Autodesk Inventor part; units mm, degrees
ref_plane "YZ Plane" through (0, 0, 0) normal (1, 0, 0) x (0, 1, 0)
ref_plane "XZ Plane" through (0, 0, 0) normal (0, 1, 0) x (-1, 0, 0)
ref_plane "XY Plane" through (0, 0, 0) normal (0, 0, 1) x (1, 0, 0)
sketch "Sketch1" plane through (0, 0, 0) normal (0, 0, 1) x (1, 0, 0)
  line L0 (-50, 30) -> (-50, 47.5)
  line L1 (50, 30) -> (50, 47.5)
  line L2 (-18.1144, 47.5) -> (0, 40)
  line L3 (0, 40) -> (18.1144, 47.5)
  line L4 (-100, 30) -> (-50, 30)
  line L5 (50, 30) -> (100, 30)
  line L6 (0, 40) -> (0, 46.5) construction
  line L7 (-18.1144, 47.5) -> (-50, 47.5)
  line L8 (18.1144, 47.5) -> (50, 47.5)
  line L9 (-100, 30) -> (-100, 0)
  line L10 (100, 0) -> (100, 30)
  line L11 (-100, 0) -> (0, 0)
  line L12 (0, 0) -> (100, 0)
  dimension "d90" = 17.5
  dimension "d91" = 50
  dimension "d92" = 50
  dimension "d105" = 10
  dimension "d108" = 30
  dimension "d110" = 50
  dimension "d154" = 18.1144
extrude "Extrusion1" add sketch "Sketch1" against normal blind 780
sketch "Sketch4" plane through (-100, 30, 0) normal (0, 1, 0) x (1, 0, 0)
  line L0 (0, 0) -> (0, 780)
  line L1 (50, 0) -> (0, 0)
  line L2 (200, 0) -> (200, 780)
  line L3 (200, 0) -> (150, 0)
  point P0 (100, 0)
  point P1 (30, 110.7)
  point P2 (170, 110.7)
  dimension "d63" = 30
  dimension "d64" = 110.7
  dimension "d65" = 30
  dimension "d109" = 110.7
hole "Hole2" at (-70, 30, -110.7) at (70, 30, -110.7) direction (0, -1, 0) diameter 15.875 depth 20 tip angle 137
thread "Thread1"
thread "Thread2"
chamfer "Chamfer1" distance 1 angle 45 4 edges at (-50, 47.5, -390) (-100, 30, -390) (50, 47.5, -390) (100, 30, -390)
sketch "Sketch6" plane through (-100, 0, 0) normal (0, -1, 0) x (1, 0, 0)
  line L0 (190, -60) -> (190, -115.207) construction
  line L1 (190, -60) -> (167.102, -60) construction
  line L2 (167.102, -60) -> (167.102, -115.207) construction
  line L3 (100, 0) -> (100, -780) construction
  line L4 (10, -60) -> (10, -115.207) construction
  line L5 (10, -60) -> (32.898, -60) construction
  line L6 (32.898, -60) -> (32.898, -115.207) construction
  line L7 (200, -390) -> (0, -390) construction
  line L8 (0, 0) -> (0, -780) construction
  line L9 (190, -720) -> (190, -664.793) construction
  line L10 (190, -720) -> (167.102, -720) construction
  line L11 (167.102, -720) -> (167.102, -664.793) construction
  line L12 (10, -720) -> (10, -664.793) construction
  line L13 (32.898, -720) -> (32.898, -664.793) construction
  line L14 (10, -720) -> (32.898, -720) construction
  line L15 (0, 0) -> (200, 0) construction
  line L16 (200, 0) -> (200, -780)
  dimension "d112" = 55.207
  dimension "d113" = 22.898
  dimension "d115" = 60
  dimension "d155" = 10
hole "Hole3" at (90, 0, -60) at (90, 0, -115.207) at (67.102, 0, -60) at (67.102, 0, -115.207) at (-90, 0, -60) at (-90, 0, -115.207) at (-67.102, 0, -60) at (-67.102, 0, -115.207) at (90, 0, -720) at (90, 0, -664.793) at (67.102, 0, -720) at (67.102, 0, -664.793) at (-67.102, 0, -720) at (-67.102, 0, -664.793) at (-90, 0, -720) at (-90, 0, -664.793) direction (0, 1, 0) diameter 4.917 depth 17.1 tip angle 137
sketch "Sketch8" plane through (0, 0, -780) normal (0, 0, -1) x (-1, 0, 0)
  line L0 (-100, 29) -> (-100, 0)
  line L1 (-100, 0) -> (100, 0)
  line L2 (0, 40) -> (-18.1144, 47.5)
  line L3 (18.1144, 47.5) -> (0, 40)
  point P0 (0, 0)
  point P1 (0, 20)
  dimension "d156" = 100
  dimension "d157" = 20
hole "Hole4" at (0, 20, -780) direction (0, 0, 1) diameter 14.376 depth 35 tip angle 137
equation "\"d92\" = d91"
equation "\"d36\" = d34"
properties part number "Base soporte tubos" material "Steel AISI 1045 HV HR"
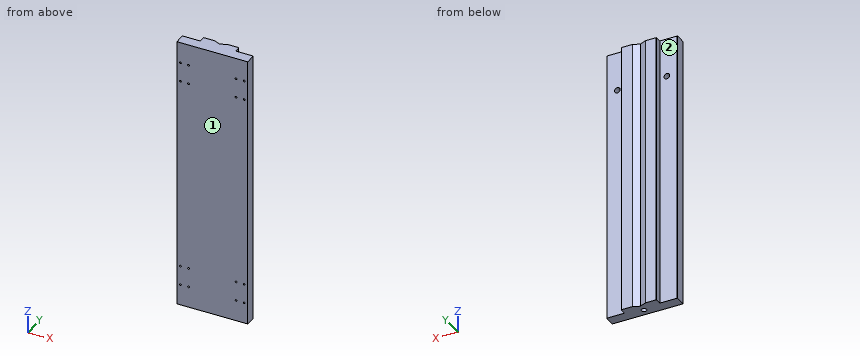
Here's how the part is built. I have some questions about the finished solid (model axes, mm). Face numbers are marked on the shaded views. A direction names the side the tool comes from. Give positions to 0.01 mm unless a question says otherwise; leave off trailing zeros. Write each loop counter-clockwise with the first axis right and the second up, starting at its lowest first coordinate (ties: lowest second). Pieces come first, ordered by that corner, then holes. Notation, with made-up numbers: (35, -26.75) -> (61, -26.75) arc R22 ccw to (61, 8.25) -> close; hole circle Ø4 at (-35, 6). An arc over 180 degrees is marked (long way). Write each question's results on one line, items separated by ' | '.
Item 1: Suppose I cut it at A-A on z = -178.5. Write out the boundary of the cut face in (x, y).
Output:
outline: (-100, 0) -> (100, 0) -> (100, 29) -> (99, 30) -> (50, 30) -> (50, 46.5) -> (49, 47.5) -> (18.11, 47.5) -> (0, 40) -> (-18.11, 47.5) -> (-49, 47.5) -> (-50, 46.5) -> (-50, 30) -> (-99, 30) -> (-100, 29) -> close
Item 2: If I drill on L1, parallel to Z at x = -90, y = 7.75; L2, parallel to X at y = 12, z = -60; L3, parallel to Z at x = -70, y = 23.5, over which ranges is the centre line in solid material (lowest first)?
Output:
L1: z = -780 to -722.46, -717.54 to -667.25, -662.33 to -117.67, -112.75 to -62.46, -57.54 to 0 | L2: x = -100 to -92.46, -87.54 to -69.56, -64.64 to 64.64, 69.56 to 87.54, 92.46 to 100 | L3: z = -780 to -118.64, -102.76 to 0
Item 3: For pin 1 Ø1.5 at (y, z) = (37.5, -673) entering from +X; pin 2 Ø8 at (x, z) = (-90, -664.793) entering from +Y; pin 3 Ø1.5 at (y, z) = (35.5, -123.5) entering from -X; pin 4 Ø12 at (x, z) = (-62, -299) entering from -Y, each with a flat end and sliding along its axis, tell me the tip position at first contact or that it passes through.
Output:
pin 1: stops at x = 50 | pin 2: stops at y = 30 | pin 3: stops at x = -50 | pin 4: stops at y = 0
Item 4: On a 3-axis mill with a long thin cutter (end or side, diameter ignored), from which of +Z, -Z, +X, -X, +Y, -Y can I reach the whole of each face in a straight line? I mean the marked faces 1 and 2. Say none if no direction works.
Output:
face 1: +Z, -Z, +X, -X, -Y | face 2: +Z, -Z, -X, +Y
